```python
from build123d import *

# Parameters (mm, degrees)
PAD_DEPTH          = 5.1
POCKET_DEPTH       = 0.5
POLARPATTERN_COUNT = 4


with BuildPart() as part:
    # Sketch → Pad (new body)
    with BuildSketch(Plane.XY):
        Polygon((8.8, -6), (8.8, 6), (6, 8.8), (-6, 8.8), (-8.8, 6), (-8.8, -6), (-6, -8.8), (6, -8.8), align=None)
    extrude(amount=PAD_DEPTH)

    # Sketch002 (on Face7 of Pad) → Pocket (cut)
    with BuildSketch(Plane.XZ.offset(8.8)):
        Polygon((-3, 5.1), (-3, 4.1), (-5, 4.1), (-5, 5.1), (-6, 5.1), (-6, 3.1), (-2, 3.1), (-2, 5.1), align=None)
        Polygon((-1, 5.1), (-1, 3.6), (-0.5, 3.1), (0.5, 3.1), (1, 3.6), (1, 5.1), align=None)
        Polygon((2, 5.1), (2, 3.1), (6, 3.1), (6, 5.1), (5, 5.1), (5, 4.1), (3, 4.1), (3, 5.1), align=None)
    pocket = extrude(amount=-POCKET_DEPTH, mode=Mode.SUBTRACT)

    # PolarPattern: Pocket ×4 about axis
    polarpattern_axis = Axis((0, 0, 0), (0, 0, 1))
    for i in range(1, POLARPATTERN_COUNT):
        add(pocket.rotate(polarpattern_axis, i * 360 / POLARPATTERN_COUNT), mode=Mode.SUBTRACT)


solid = part.part
```
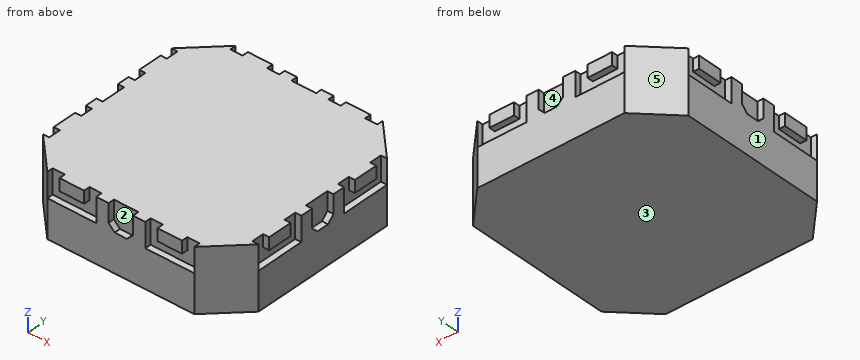
Geometry check sheet. Reference: the model listing, model coordinates, mm. Face numbers are marked on the shaded views. A direction names the side the tool comes from. Give positions to 0.01 mm unless a question says otherwise; leave off trailing zeros. Order: outer loops, then holes, each group sorted by start corner. A loop starts at its lowest first (then second) coordinate and runs counter-clockwise, first axis right, second up. Notation, with made-up numbers: (32, 57.5) - (71, 57.5) arc R20 ccw to (71, 65.5) - close; hole circle Ø1 at (61.5, 53). An arc over 180 degrees is marked (long way). Answer in a Markdown table with one row per item. Add a question column.
Q1. Mould release check, pull along X, two halves, no side actions. Record for the marked faces 1, 2 and 3: pulls with the +X half, pulls with the -X half, needs draft (parallel to the pull), parting line crosses it, or undercut.
Q2. Tool access check on the marked faces 4 and 5. Record the directions out of +Z, -Z, +X, -X, +Y, -Y that give a thin tool (end or side, any length) a straight path to the whole face; none if there is none.
Q3. Material ranges on probe 1 along X at (y, z) = (-0.75, 4.05); probe 2 along X at (y, z) = (-7.5, 0.5), recorded low to high. Write a range as from..to.
Q4. Cross-section at B-B, the plane z = 2.5. Enter the section's corners in (x, y), then the cut area to 3 significant figures.
Q5. Gauge pin test, flat ends, axial feed: pin 1 (0.6 mm diameter, centred on x = 8.5, z = 4.5, fed in from -Y); pin 2 (0.6 mm diameter, centred on x = 8.5, z = 4.5, fed in from +Y). Record the tip position at first contact, or that the pin passes through.
Q6. Cross-section at A-A, the plane x = -5.75. Enter the section's corners in (y, z).
Check values:
| question | item | result |
|---|---|---|
| 1 | face 1 | pulls with the -X half |
| 1 | face 2 | undercut |
| 1 | face 3 | needs draft |
| 2 | face 4 | +Z, +Y |
| 2 | face 5 | +Z, -Z, -X, +Y |
| 3 | probe 1 | x = -8.3..8.3 |
| 3 | probe 2 | x = -7.3..7.3 |
| 4 | outline | (-8.8, -6) - (-6, -8.8) - (6, -8.8) - (8.8, -6) - (8.8, 6) - (6, 8.8) - (-6, 8.8) - (-8.8, 6) - close |
| 4 | area | 294 mm^2 |
| 5 | pin 1 | stops at y = -6.6 |
| 5 | pin 2 | stops at y = 6.6 |
| 6 | outline | (-8.8, 0) - (8.8, 0) - (8.8, 3.1) - (8.3, 3.1) - (8.3, 5.1) - (-8.3, 5.1) - (-8.3, 3.1) - (-8.8, 3.1) - close |
